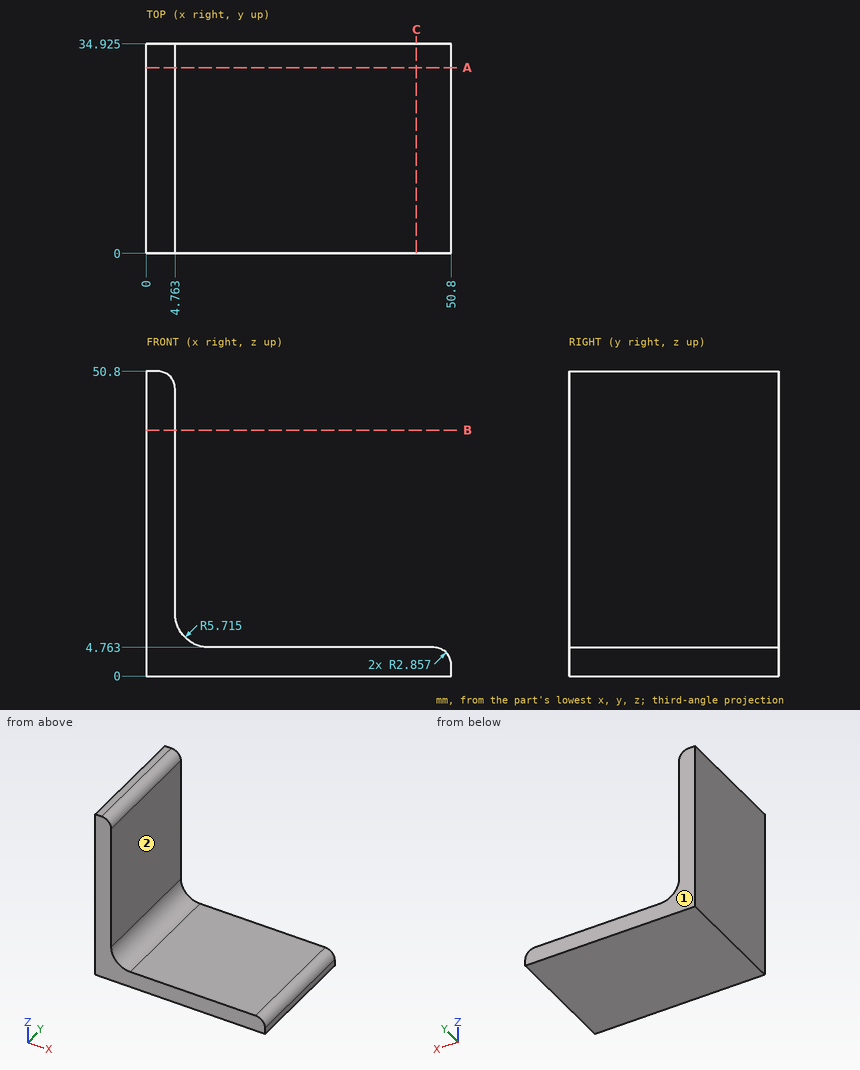
Geometry check sheet. Reference: drawing and pictorial views, mm from the part's lowest x, y, z. A direction names the side the tool comes from. Give positions to 0.01 mm unless a question says otherwise; leave off trailing zeros. Loops run counter-clockwise (first coordinate to the right, second up) from the corner with the lowest first, then second, coordinate; pieces in that order, holes last.
1. Section check B-B, the plane z = 41. Enter the section's corners in (x, y) (1 decimal), then the cut area to 3 significant figures.
2. Section check C-C, the plane x = 45. Enter the section's corners in (y, z) (1 decimal), then the cut area to 3 significant figures.
3. Set-up check for the marked faces 1 and 2: record each of +Z, -Z, +X, -X, +Y, -Y from which the full face is reachable in a straight line by a thin tool's end or side.
4. Thickness scan on line 1 (Z direction, x = 11, y = 2); line 2 (Z direction, x = 8, y = 23). Record the ranges inside material, lowest first.
5. Go/stop test with flat-tipped pins: pin 1 Ø6 at (y, z) = (26, 37.5) entering from +X; pin 2 Ø1 at (x, y) = (35, 27) entering from +Z. Record where each tip stops, or that it passes through.
6. Section check A-A, the plane y = 31. Enter the section's corners in (x, z) (1 decimal).
Geometry says:
1. outline: (0, 0) - (4.8, 0) - (4.8, 34.9) - (0, 34.9) - close
1. area: 166 mm2
2. outline: (0, 0) - (34.9, 0) - (34.9, 4.8) - (0, 4.8) - close
2. area: 166 mm2
3. face 1: +Z, -Z, +X, -X, +Y
3. face 2: +Z, +X, +Y, -Y
4. line 1: z = 0 to 4.76
4. line 2: z = 0 to 5.33
5. pin 1: stops at x = 4.76
5. pin 2: stops at z = 4.76
6. outline: (0, 0) - (50.8, 0) - (50.8, 1.9) arc R2.9 ccw to (47.9, 4.8) - (10.5, 4.8) arc R5.7 cw to (4.8, 10.5) - (4.8, 47.9) arc R2.9 ccw to (1.9, 50.8) - (0, 50.8) - close
